Work out the finished part from the listing and answer in its coordinate system (mm). Face numbers are marked on the shaded views. A direction names the side the tool comes from. Coordinates: 2 decimals unless noted, no trailing zeros. Order: outer loops, then holes, each group sorted by start corner. A loop starts at its lowest first (then second) coordinate and runs counter-clockwise, first axis right, second up. Notation, with made-up numbers: (-4.75, 38.25) - (13.25, 38.25) arc R11 cw to (13.25, 43.25) - close; hole circle Ø6 at (26, 80.25). An arc over 180 degrees is marked (long way). Use CSV: the item, a comma, the result in double quotes. Start each with the question number.
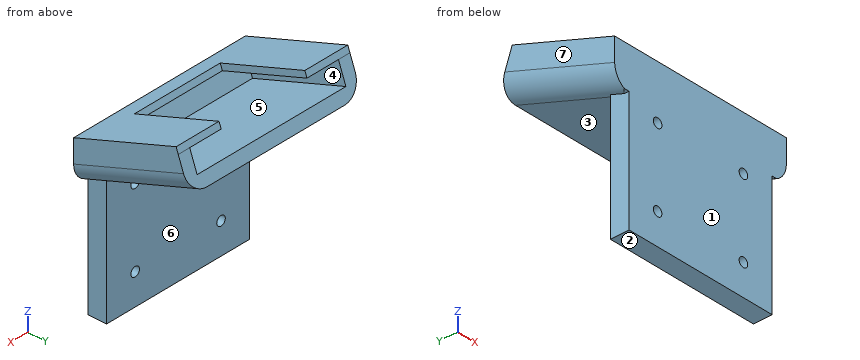
Autodesk Inventor part; units mm, degrees
ref_plane "Work Plane1" through (-12.5, 3, 11.25) normal (0, -0.3420201, 0.9396926) x (1, 0, 0)
ref_plane "YZ Plane" through (0, 0, 0) normal (1, 0, 0) x (0, 1, 0)
ref_plane "XZ Plane" through (0, 0, 0) normal (0, 1, 0) x (-1, 0, 0)
sketch "Sketch1" plane through (0, 0, 0) normal (0, 1, 0) x (-1, 0, 0)
  line L0 (12.5, 11.25) -> (-12.5, 11.25)
  line L1 (-12.5, 11.25) -> (-12.5, -11.25)
  line L2 (-12.5, -11.25) -> (12.5, -11.25)
  line L3 (12.5, -11.25) -> (12.5, 11.25)
  line L4 (12.5, 11.25) -> (-12.5, -11.25) construction
  line L5 (-12.5, 11.25) -> (12.5, -11.25) construction
  line L6 (7.5, 6.25) -> (-7.5, 6.25) construction
  line L7 (-7.5, 6.25) -> (-7.5, -6.25) construction
  line L8 (-7.5, -6.25) -> (7.5, -6.25) construction
  line L9 (7.5, -6.25) -> (7.5, 6.25) construction
  line L10 (7.5, 6.25) -> (-7.5, -6.25) construction
  line L11 (-7.5, 6.25) -> (7.5, -6.25) construction
  circle A0 centre (7.5, -6.25) radius 0.75
  circle A1 centre (-7.5, -6.25) radius 0.75
  circle A2 centre (-7.5, 6.25) radius 0.75
  circle A3 centre (7.5, 6.25) radius 0.75
  point P0 (0, 0)
  dimension "d0" = 12.5
  dimension "d1" = 15
  dimension "d2" = 5
  dimension "d3" = 5
  dimension "d4" = 1.5
  dimension "d5" = 1.5
  dimension "d6" = 1.5
  dimension "d7" = 1.5
extrude "Extrusion1" add sketch "Sketch1" along normal blind 3
ref_plane "Work Plane1" through (-12.5, 3, 11.25) normal (0, -0.3420201, 0.9396926) x (1, 0, 0)
sketch "Sketch2" plane through (-12.5, 3, 11.25) normal (0, -0.3420201, 0.9396926) x (1, 0, 0)
  line L0 (0, -7.6955) -> (0, 0) construction
  line L1 (25, 0) -> (25, -7.6955) construction
  line L2 (0, 0) -> (25, 0) construction
  line L3 (-2.5, 16) -> (27.5, 16)
  line L4 (27.5, 16) -> (27.5, -3)
  line L5 (27.5, -3) -> (-2.5, -3)
  line L6 (-2.5, -3) -> (-2.5, 16)
  line L7 (-2.5, 16) -> (27.5, -3) construction
  line L8 (27.5, 16) -> (-2.5, -3) construction
  point P0 (12.5, -6.6668)
  point P1 (12.5, 6.5)
  point P2 (12.5, 0)
  dimension "d11" = 19
  dimension "d12" = 16
  dimension "d13" = 30
extrude "Extrusion2" add sketch "Sketch2" against normal blind 2
sketch "Sketch3" plane through (-12.5, 3, 11.25) normal (0, -0.3420201, 0.9396926) x (1, 0, 0)
  line L0 (0, 0) -> (25, 0) construction
  line L1 (-0.5, 0) -> (25.5, 0) construction
  line L2 (25.5, 0) -> (25.5, 16) construction
  line L3 (25.5, 16) -> (-0.5, 16) construction
  line L4 (-0.5, 16) -> (-0.5, 0) construction
  line L5 (-0.5, 0) -> (25.5, 16) construction
  line L6 (25.5, 0) -> (-0.5, 16) construction
  line L7 (-2.5, -3) -> (-2.5, 16) construction
  line L8 (-0.5, 16) -> (-2.5, 16)
  line L9 (-2.5, 16) -> (-2.5, 0)
  line L10 (-2.5, 0) -> (-0.5, 0)
  line L11 (-0.5, 0) -> (-0.5, 16)
  line L12 (27.5, 16) -> (27.5, -3) construction
  line L13 (25.5, 16) -> (27.5, 16)
  line L14 (27.5, 16) -> (27.5, 0)
  line L15 (27.5, 0) -> (25.5, 0)
  line L16 (25.5, 0) -> (25.5, 16)
  line L17 (-2.5, 0) -> (27.5, 0)
  line L18 (27.5, 0) -> (27.5, -2)
  line L19 (27.5, -2) -> (-2.5, -2)
  line L20 (-2.5, -2) -> (-2.5, 0)
  point P0 (12.5, -6.6668)
  point P1 (12.5, 8)
  point P2 (12.5, 0)
  point P3 (-0.5, 0)
  dimension "d16" = 16
  dimension "d17" = 26
  dimension "d18" = 2
extrude "Extrusion3" add sketch "Sketch3" along normal blind 3.5
sketch "Sketch4" plane through (-12.5, 1.8029, 14.5389) normal (0, -0.3420201, 0.9396926) x (1, 0, 0)
  line L0 (-2.5, 16) -> (-2.5, -2)
  line L1 (-2.5, -2) -> (27.5, -2)
  line L2 (27.5, -2) -> (27.5, 16)
  line L3 (27.5, 16) -> (25.5, 16) construction
  line L4 (-0.5, 16) -> (-2.5, 16) construction
  line L5 (-2.5, -2) -> (27.5, -2) construction
  line L6 (27.5, -2) -> (27.5, 16) construction
  line L7 (27.5, 16) -> (-2.5, 16)
  line L8 (-2.5, 16) -> (-2.5, -2) construction
  line L9 (5, 1.5) -> (20, 1.5)
  line L10 (20, 1.5) -> (20, 16)
  line L11 (20, 16) -> (5, 16)
  line L12 (5, 16) -> (5, 1.5)
  line L13 (5, 1.5) -> (20, 16) construction
  line L14 (20, 1.5) -> (5, 16) construction
  point P0 (12.5, -6.6668)
  point P1 (12.5, 8.75)
  point P2 (12.5, 16)
  point P3 (20, 16)
  dimension "d21" = 15
  dimension "d23" = 3.5
extrude "Extrusion4" add sketch "Sketch4" along normal blind 1 contours L7 L12 L9 L10 L2 L1 L0
sketch "Sketch5" plane through (12.5, 1.1206, 10.566) normal (0, -0.9396926, -0.3420201) x (1, 0, 0)
  line L0 (2.5, 0) -> (2.5, 4.5)
  line L1 (0, 0) -> (0, 0.7279)
  line L2 (2.5, 0) -> (0, 0)
  line L3 (-27.5, 4.5) -> (2.5, 4.5)
  line L4 (0, 0.7279) -> (-25, 0.7279)
  line L5 (-25, 0) -> (-27.5, 0)
  line L6 (-27.5, 0) -> (-27.5, 4.5)
  line L7 (-25, 0.7279) -> (-25, 0)
  point P0 (-12.5, -9.5455)
extrude "Extrusion5" add sketch "Sketch5" along normal blind 1
sketch "Sketch6" plane through (12.5, 0.865, 8.3446) normal (0, -0.9396926, -0.3420201) x (1, 0, 0)
  line L0 (2.5, 0) -> (0, 0)
  line L1 (-25, 2.7279) -> (0, 2.7279)
  line L2 (-25, 0) -> (-27.5, 0)
  line L3 (2.5, 0) -> (-27.5, 0)
  line L4 (-27.5, 0) -> (-27.5, 2.7279)
  line L5 (-27.5, 2.7279) -> (2.5, 2.7279)
  line L6 (2.5, 2.7279) -> (2.5, 0)
  point P0 (-12.5, -7.5455)
  point P1 (-25, 0)
  point P2 (0, 0)
  point P3 (0, 2.7279)
sketch3d "3D Sketch1"
  line L0 (12.5, 3, -11.25) -> (12.5, 0, -11.25)
sweep "Sweep1" add profiles "Sketch6" path "3D Sketch1"
sketch "Sketch7" plane through (12.5, 0, -11.25) normal (0, 0, -1) x (-1, 0, 0)
  line L0 (-2.5, 0) -> (27.5, 0)
  line L1 (27.5, 0) -> (27.5, -3.068)
  line L2 (27.5, -3.068) -> (-2.5, -3.068)
  line L3 (-2.5, -3.068) -> (-2.5, 0)
  line L4 (0, 0) -> (25, 0)
  line L5 (27.5, 0.865) -> (27.5, -2.135)
  line L6 (-2.5, 0.865) -> (-2.5, -2.135)
  line L7 (-2.5, -3.068) -> (27.5, -3.068)
  point P0 (12.5, 0)
extrude "Extrusion6" cut sketch "Sketch7" against normal through all
fillet "Fillet1" radius 3 2 edges at (15, 9.792, 11.5937) (-15, 9.792, 11.5937)
equation "\"d5\" = d4"
equation "\"d6\" = d4"
equation "\"d7\" = d4"
properties part number "camera-mount"
1) For the marked faces 5, 6 and 7, determine the directions among +Z, -Z, +X, -X, +Y, -Y from which every point of the face is accessible in a straight line to the end or side of a thin tool.
2) Straight lines are drawn through the part: line 1 (Z direction, x = 7.5, y = 1.05); line 2 (Z direction, x = -7.5, y = 1.75); line 3 (Y direction, x = -2.5, z = -2). For each, find the intervals that lie inside material, in ascending order. Write a range as [from, to].
3) The part is cut by section C-C on x = -11.5. Determine the outline of the cut face in (y, z), plus the area to 3 significant figures.
4) Flat-ended cylindrical pins translate along their axes: P1, Ø0.9, axis at y = 2, z = 0, coming from the +X side; P2, Ø2.5, axis at x = -7.5, z = 6.25, coming from the +Y side; P3, Ø10, axis at x = -3, y = 9, coming from the +Z side. Find the tip coordinate at first contact, or state that the pin passes through.
5) For a pull along Y with two mould halves and no side action, classify the marked faces 1, 2, 3 and 4 as +Y half, -Y half, draft (parallel to the pull), parting line (faces both ways), or undercut.
6) The part is cut by section A-A on z = -6.25. Determine the outline of the cut face in (x, y), plus the area to 3 significant figures.
7) The part is cut by section B-B on x = -5.75. Determine the outline of the cut face in (y, z).
Answer key:
1,face 5,"none"
1,face 6,"-Z, +X, -X, +Y"
1,face 7,"+Z, -Z, -X, +Y, -Y"
2,line 1,"[-11.25, -7], [-5.5, 5.5], [7, 15.33]"
2,line 2,"[-11.25, -7], [-5.5, 5.5], [7, 15.58]"
2,line 3,"[0, 3]"
3,outline,"(0, -11.25) - (3, -11.25) - (3, 9.12) - (18.72, 14.84) - (18.04, 16.72) - (3, 11.25) - (1.8, 14.54) - (16.84, 20.01) - (16.5, 20.95) - (0, 14.95) - close"
3,area,"125 mm^2"
4,P1,"x = 12.5"
4,P2,"y = 3"
4,P3,"z = 19.02"
5,face 1,"-Y half"
5,face 2,"draft"
5,face 3,"+Y half"
5,face 4,"undercut"
6,outline,"(-12.5, 0) - (-8.25, 0) - (-8.25, 3) - (-12.5, 3) - close; (-6.75, 0) - (6.75, 0) - (6.75, 3) - (-6.75, 3) - close; (8.25, 0) - (12.5, 0) - (12.5, 3) - (8.25, 3) - close"
6,area,"66.0 mm^2"
7,outline,"(0, -11.25) - (3, -11.25) - (3, 9.12) - (18.72, 14.84) - (18.04, 16.72) - (3, 11.25) - (1.8, 14.54) - (3.21, 15.05) - (2.87, 15.99) - (0, 14.95) - close"
